from build123d import *

# Parameters (mm, degrees)
CHAMFER1_SIZE  = 1
CHAMFER1_SIZE2 = 2.246036774


with BuildPart() as part:
    # Sketch1 → Revolve1 (revolve)
    with BuildSketch(Plane.XY):
        Polygon((0, 0), (4.5, 0), (5.75, 8.5), (5.75, 22.3), (7, 22.3), (8.25, 22.55), (8.25, 24.05), (7, 24.3), (5.75, 24.3), (5.75, 37.3), (0, 37.3), align=None)
    revolve(axis=Axis((0, -143.950460456, 0), (0, 1, 0)))

    # Sketch2 → Cut-Revolve1 (revolve, cut)
    with BuildSketch(Plane.XY):
        Polygon((1.1, 0), (1.1, 2), (2.5, 2), (2.5, 14.18), (3.5, 14.18), (3.5, 37.3), (0, 37.3), (0, 0), align=None)
    revolve(axis=Axis((0, -1000, 0), (0, 1, 0)), mode=Mode.SUBTRACT)

    # Chamfer1
    chamfer1_edges = [part.edges().sort_by_distance(p)[0] for p in [
        (-2.5, 2, 0),
    ]]
    chamfer1_side = [part.faces().sort_by_distance(p)[0] for p in [
        (-1.170710678, 2, 0),
    ]]
    chamfer(chamfer1_edges, length=CHAMFER1_SIZE, length2=CHAMFER1_SIZE2, reference=chamfer1_side[0])


solid = part.part
Design review of the part built by this model. Coordinates are the model's own, in mm. A direction names the side the tool comes from. Coordinates: 2 decimals unless noted, no trailing zeros. Write each loop counter-clockwise with the first axis right and the second up, starting at its lowest first coordinate (ties: lowest second). Pieces come first, ordered by that corner, then holes. Notation, with made-up numbers: (-28, 13.5) -> (10, 13.5) arc R16 ccw to (10, 43.5) -> close; hole circle Ø9 at (57, 66). An arc over 180 degrees is marked (long way). Write each question's results on one line, items separated by ' | '. Start each with the question number.
(1) Tool access review of faces 1 (the face through (-0.54, 9.28, 2.44)), 2 (the face through (0, 37.3, 4)): name each direction out of +Z, -Z, +X, -X, +Y, -Y from which nothing blocks a thin tool from reaching the whole face with its end or side.
(2) For line 1 along Z through (x, y) = (0, 10); line 2 along X through (y, z) = (18, 0), list the stretches that pass through material, from the lowest coordinate up. Write a range as from..to.
(3) The part is to be moulded in two halves that separate along Z. For faces 3 (the face through (1.05, 1.01, -0.33)), 4 (the face through (1, 22.3, -6)), 5 (the face through (-0.75, 15.5, -5.7)), say which applies: pulls with the +Z half, pulls with the -Z half, needs draft (parallel to the pull), parting line crosses it, or undercut.
(4) Clearance check with flat-ended pins moving along their axes: P1, Ø5, axis at x = 3, y = 6, coming from the -Z side; P2, Ø1, axis at x = -4.5, y = 5.5, coming from the -Z side; P3, Ø2.5, axis at x = -0.5, z = -0.5, coming from the +Y side. State where each tip first meets the part, or that it passes through.
(5) Take a section at C-C on y = 5. Write out the cut boundary in (x, z), and give its area (3 significant figures).
Results found:
1) face 1: +Y | face 2: +Z, -Z, +X, -X, +Y
2) line 1: z = -5.75..-2.5, 2.5..5.75 | line 2: x = -5.75..-3.5, 3.5..5.75
3) face 3: undercut | face 4: needs draft | face 5: parting line crosses it
4) P1: stops at z = -5.51 | P2: stops at z = -3.5 | P3: stops at y = 3.03
5) outline: circle Ø10.47 at (0, 0); hole circle Ø5 at (0, 0) | area: 66.5 mm2
